from build123d import *

# Parameters (mm, degrees)
EXTRUDE_1_DEPTH          = 200
CUT_EXTRUDE_1_DEPTH      = 193.621587163
CUT_EXTRUDE_1_DEPTH_BACK = 193.621587163
CUT_EXTRUDE_2_DEPTH      = 192.309050473
CUT_EXTRUDE_2_DEPTH_BACK = 192.309050473
SKETCH_8_R               = 2
CUT_EXTRUDE_3_DEPTH      = 192.309050473
CUT_EXTRUDE_3_DEPTH_BACK = 192.309050473
SKETCH_9_W               = 52
SKETCH_9_H               = 25


with BuildPart() as part:
    # 草图5 → 凸台-拉伸1 (new body)
    with BuildSketch(Plane(origin=(-52, 0, 0), x_dir=(-0.8660254037844397, 0, -0.4999999999999983), z_dir=(0.4999999999999982, 0, -0.8660254037844396))):
        with BuildLine():
            Line((-11, -15), (11, -15))
            ThreePointArc((11, -15), (13.828427125, -13.828427125), (15, -11))
            Line((15, -11), (15, 11))
            ThreePointArc((15, 11), (13.828427125, 13.828427125), (11, 15))
            Line((11, 15), (-11, 15))
            ThreePointArc((-11, 15), (-13.828427125, 13.828427125), (-15, 11))
            Line((-15, 11), (-15, -11))
            ThreePointArc((-15, -11), (-13.828427125, -13.828427125), (-11, -15))
        make_face()
        with BuildLine():
            Line((-11, -13), (11, -13))
            ThreePointArc((11, -13), (12.414213562, -12.414213562), (13, -11))
            Line((13, -11), (13, 11))
            ThreePointArc((13, 11), (12.414213562, 12.414213562), (11, 13))
            Line((11, 13), (-11, 13))
            ThreePointArc((-11, 13), (-12.414213562, 12.414213562), (-13, 11))
            Line((-13, 11), (-13, -11))
            ThreePointArc((-13, -11), (-12.414213562, -12.414213562), (-11, -13))
        make_face(mode=Mode.SUBTRACT)
    extrude(amount=EXTRUDE_1_DEPTH)

    # 草图7 → 切除-拉伸1 (cut, two sides: drawn at the far end of the back side and taken through both)
    with BuildSketch(Plane(origin=(0, 0, 0), x_dir=(1, 0, 0), z_dir=(0, 1, 0)).offset(-CUT_EXTRUDE_1_DEPTH_BACK)):
        Polygon((2.851111613, -65.004912165), (-65.527886261, 53.430986323), (-91.508648375, 38.430986323), (-23.129650501, -80.004912165), align=None)
    extrude(amount=CUT_EXTRUDE_1_DEPTH + CUT_EXTRUDE_1_DEPTH_BACK, mode=Mode.SUBTRACT)

    # 草图8 → 切除-拉伸2 (cut, two sides: drawn at the far end of the back side and taken through both)
    with BuildSketch(Plane(origin=(0, 0, 0), x_dir=(1, 0, 0), z_dir=(0, 1, 0)).offset(-CUT_EXTRUDE_2_DEPTH_BACK)):
        with Locations(Location((-26, 45.033320997, 0), (0, 0, 270))):
            Circle(SKETCH_8_R)
        with Locations(Location((16.614746246, 118.844226646, 0), (0, 0, 270))):
            Circle(SKETCH_8_R)
    extrude(amount=CUT_EXTRUDE_2_DEPTH + CUT_EXTRUDE_2_DEPTH_BACK, mode=Mode.SUBTRACT)

    # 草图9 → 切除-拉伸3 (cut, two sides: drawn at the far end of the back side and taken through both)
    with BuildSketch(Plane(origin=(0, 0, 0), x_dir=(1, 0, 0), z_dir=(0, 1, 0)).offset(-CUT_EXTRUDE_3_DEPTH_BACK)):
        with Locations((0, 17.533320997)):
            Rectangle(SKETCH_9_W, SKETCH_9_H)
    extrude(amount=CUT_EXTRUDE_3_DEPTH + CUT_EXTRUDE_3_DEPTH_BACK, mode=Mode.SUBTRACT)


solid = part.part
Design review of the part built by this model. Coordinates are the model's own, in mm. A direction names the side the tool comes from. Coordinates: 2 decimals unless noted, no trailing zeros. Write each loop counter-clockwise with the first axis right and the second up, starting at its lowest first coordinate (ties: lowest second). Pieces come first, ordered by that corner, then holes. Notation, with made-up numbers: (37, 56.5) - (86, 56.5) arc R27 cw to (86, 81.5) - close; hole circle Ø1 at (-20, 79). An arc over 180 degrees is marked (long way). One line per item, written item: value.
1) Mouldability with a two-part tool opening along X and no side actions: class faces 1 (the face through (-8.7, 13.8, -102.71)), 2 (the face through (-27.22, 13.99, -46.62)), 3 (the face through (-19, 0, -30.033)) as +X half, -X half, draft (parallel to the pull), parting line (faces both ways), or undercut.
Answer sheet:
face 1: -X half
face 2: undercut
face 3: draft
2) To check wall thickness, follow probe 1 along Y at (x, z) = (-14, -62); probe 2 along Z at (x, y) = (-12, -12); probe 3 along X at (y, z) = (-6, -160). State the ranges of each line that lie inside material, in increasing order.
Answer sheet:
probe 1: y = -15 to -13, 13 to 15
probe 2: z = -99.03 to -94.75, -43.82 to -39.54
probe 3: x = 23.06 to 25.36, 55.39 to 57.7
3) For faces 4 (the face through (-9.104, -0.154, -104.298)), 5 (the face through (-30.63, -12.4, -12.16)), 6 (the face through (19.25, 0.15, -97.41)), list the 3-axis set-ups (+Z, -Z, +X, -X, +Y, -Y) from which the entire face can be reached by the end or side of a thin tool; tool diameter is ignored.
Answer sheet:
face 4: -Z, -X, +Y, -Y
face 5: -X
face 6: none
4) Insertion check: pin 1 (7 mm diameter, centred on x = -19.5, y = -4.5, fed in from +Z); pin 2 (3 mm diameter, centred on y = 9.5, z = -51, fed in from +X); pin 3 (10 mm diameter, centred on y = 11, z = -76.5, fed in from -X). Each pin has a flat end and moves straight along its axis. Give the tip position at first contact, or say it passes through.
Answer sheet:
pin 1: stops at z = -30.03
pin 2: stops at x = -4.37
pin 3: stops at x = -28.04
5) Add section A-A (y = 7). State the section outline as (x, z) points, plus the area to 3 significant figures.
Answer sheet:
outline: (-52, -30) - (35.01, -180.71) - (36.74, -179.71) - (-50.85, -28) - close; (-35.83, -2) - (-26, -19.03) - (-26, -15.03) - (-34.68, 0) - close; (-19.65, -30.03) - (59.26, -166.71) - (60.99, -165.71) - (-17.34, -30.03) - close
area: 701 mm2
